The listing builds one solid part. Answer for the finished solid, in the listing's coordinates (mm). A direction names the side the tool comes from. Give positions to 0.01 mm unless a question says otherwise; leave off trailing zeros. Write each loop counter-clockwise with the first axis right and the second up, starting at its lowest first coordinate (ties: lowest second). Pieces come first, ordered by that corner, then holes. Notation, with made-up numbers: (-32, 86) - (20, 86) arc R18 cw to (20, 115) - close; hole circle Ø11 at (-39.5, 65). An arc over 180 degrees is marked (long way). Answer as CSV lines item,"result". Start each with the question number.
(1) Find section B-B (y = 3). Write down the section's boundary in (x, z).
(2) Find section C-C (z = 26.5). Write down the section's boundary in (x, y), then the cut area to 3 significant figures.
(3) For faces 1 (the face through (6.003, 6.459, -38.794)), 2 (the face through (-25, -23, -50)), 3 (the face through (-32.5, -25, 42)), determine the directions among +Z, -Z, +X, -X, +Y, -Y from which every point of the face is accessible in a straight line to the end or side of a thin tool.
(4) Find section D-D (x = -63). Write down the section's boundary in (y, z).
(5) Find section A-A (y = -23.5). State how many separate pieces and enclosed holes the cut face has, then the cut area to 3 significant figures.
(6) Straight lines are drawn through the part: probe 1 along X at (y, z) = (-28, 0); probe 2 along X at (y, z) = (-27, 0); probe 3 along Y at (x, z) = (9, 66.5). For each, find the intervals that lie inside material, in ascending order.
(7) Each of these flat-tipped pins is pushed along its axis until it touches: pin 1 Ø1 at (x, z) = (-4.5, 56.5) entering from -Y; pin 2 Ø3 at (y, z) = (-26.5, -48.5) entering from -X; pin 3 Ø1.5 at (y, z) = (-8.5, -42) entering from -X; pin 4 Ø12 at (x, y) = (-33.5, -6.5) entering from +Z. Where does it stop, or does it pass through?
(8) For a pull along Z with two mould halves and no side action, classify faces 4 (the face through (-27.5, -24, 58)), 5 (the face through (9.415, 2.673, 34.351)), 6 (the face through (-30, -24, -62.5)) as pulls with the +Z half, pulls with the -Z half, needs draft (parallel to the pull), parting line crosses it, or undercut.
from build123d import *

# Parameters (mm, degrees)
SALIENTE_EXTRUIR2_DEPTH             = 75
SALIENTE_EXTRUIR5_DEPTH             = 17
SALIENTE_EXTRUIR5_DIRECTION_2_REACH = 107.612
CROQUIS6_R                          = 3.96875
CORTAR_EXTRUIR2_DEPTH               = 20
CROQUIS16_R                         = 5.96875
CROQUIS16_R_2                       = 3.96875
CORTAR_EXTRUIR3_DEPTH               = 3
CROQUIS17_R                         = 1
CORTAR_EXTRUIR4_DEPTH               = 13


with BuildPart() as part:
    # Croquis1 → Saliente-Extruir2 (new, symmetric)
    with BuildSketch(Plane.XY):
        with BuildLine():
            ThreePointArc((-1.339745962, 5), (12.862399029, 7.937956503), (25, 0))
            Line((25, 0), (0, 0))
            Line((0, 0), (-60.621778265, -35))
            Line((-60.621778265, -35), (-70.621778265, -35))
            Line((-70.621778265, -35), (-1.339745962, 5))
        make_face()
    extrude(amount=SALIENTE_EXTRUIR2_DEPTH, both=True)

    # Croquis3 → Saliente-Extruir5 (add)
    with BuildSketch(Plane.XZ.offset(15)):
        with BuildLine():
            Line((-32.5, 4.330127019), (-32.5, 12.5))
            Line((-32.5, 12.5), (-27.5, 12.5))
            Line((-27.5, 12.5), (-27.5, 4.330127019))
            ThreePointArc((-27.5, 4.330127019), (-25, 0), (-27.5, -4.330127019))
            Line((-27.5, -4.330127019), (-27.5, -12.5))
            Line((-27.5, -12.5), (-32.5, -12.5))
            Line((-32.5, -12.5), (-32.5, -4.330127019))
            ThreePointArc((-32.5, -4.330127019), (-35, 0), (-32.5, 4.330127019))
        make_face()
        with BuildLine():
            Line((-27.5, -45.669872981), (-27.5, -37.5))
            Line((-27.5, -37.5), (-32.5, -37.5))
            Line((-32.5, -37.5), (-32.5, -45.669872981))
            ThreePointArc((-32.5, -45.669872981), (-35, -50), (-32.5, -54.330127019))
            Line((-32.5, -54.330127019), (-32.5, -62.5))
            Line((-32.5, -62.5), (-27.5, -62.5))
            Line((-27.5, -62.5), (-27.5, -54.330127019))
            ThreePointArc((-27.5, -54.330127019), (-25, -50), (-27.5, -45.669872981))
        make_face()
        with BuildLine():
            Line((-27.5, 54.330127019), (-27.5, 62.5))
            Line((-27.5, 62.5), (-32.5, 62.5))
            Line((-32.5, 62.5), (-32.5, 54.330127019))
            ThreePointArc((-32.5, 54.330127019), (-35, 50), (-32.5, 45.669872981))
            Line((-32.5, 45.669872981), (-32.5, 37.5))
            Line((-32.5, 37.5), (-27.5, 37.5))
            Line((-27.5, 37.5), (-27.5, 45.669872981))
            ThreePointArc((-27.5, 45.669872981), (-25, 50), (-27.5, 54.330127019))
        make_face()
    extrude(amount=SALIENTE_EXTRUIR5_DEPTH)

    # Saliente-Extruir5 direction 2: up to this face of the body (flat: up to its plane)
    saliente_extruir5_direction_2_end = Plane(part.part.faces().sort_by_distance((-30.310889132, -17.5, 0))[0])
    # Croquis3 → Saliente-Extruir5 direction 2 (add, up to the picked face)
    with BuildSketch(Plane.XZ.offset(15), mode=Mode.PRIVATE) as saliente_extruir5_direction_2_sk1:
        with BuildLine():
            Line((-32.5, 4.330127019), (-32.5, 12.5))
            Line((-32.5, 12.5), (-27.5, 12.5))
            Line((-27.5, 12.5), (-27.5, 4.330127019))
            ThreePointArc((-27.5, 4.330127019), (-25, 0), (-27.5, -4.330127019))
            Line((-27.5, -4.330127019), (-27.5, -12.5))
            Line((-27.5, -12.5), (-32.5, -12.5))
            Line((-32.5, -12.5), (-32.5, -4.330127019))
            ThreePointArc((-32.5, -4.330127019), (-35, 0), (-32.5, 4.330127019))
        make_face()
    saliente_extruir5_direction_2_tool1 = split(extrude(saliente_extruir5_direction_2_sk1.sketch, amount=-SALIENTE_EXTRUIR5_DIRECTION_2_REACH, mode=Mode.PRIVATE), bisect_by=saliente_extruir5_direction_2_end, keep=Keep.BOTH, mode=Mode.PRIVATE)
    # Croquis3 → Saliente-Extruir5 direction 2 (add, up to the picked face)
    with BuildSketch(Plane.XZ.offset(15), mode=Mode.PRIVATE) as saliente_extruir5_direction_2_sk2:
        with BuildLine():
            Line((-27.5, -45.669872981), (-27.5, -37.5))
            Line((-27.5, -37.5), (-32.5, -37.5))
            Line((-32.5, -37.5), (-32.5, -45.669872981))
            ThreePointArc((-32.5, -45.669872981), (-35, -50), (-32.5, -54.330127019))
            Line((-32.5, -54.330127019), (-32.5, -62.5))
            Line((-32.5, -62.5), (-27.5, -62.5))
            Line((-27.5, -62.5), (-27.5, -54.330127019))
            ThreePointArc((-27.5, -54.330127019), (-25, -50), (-27.5, -45.669872981))
        make_face()
    saliente_extruir5_direction_2_tool2 = split(extrude(saliente_extruir5_direction_2_sk2.sketch, amount=-SALIENTE_EXTRUIR5_DIRECTION_2_REACH, mode=Mode.PRIVATE), bisect_by=saliente_extruir5_direction_2_end, keep=Keep.BOTH, mode=Mode.PRIVATE)
    # Croquis3 → Saliente-Extruir5 direction 2 (add, up to the picked face)
    with BuildSketch(Plane.XZ.offset(15), mode=Mode.PRIVATE) as saliente_extruir5_direction_2_sk3:
        with BuildLine():
            Line((-27.5, 54.330127019), (-27.5, 62.5))
            Line((-27.5, 62.5), (-32.5, 62.5))
            Line((-32.5, 62.5), (-32.5, 54.330127019))
            ThreePointArc((-32.5, 54.330127019), (-35, 50), (-32.5, 45.669872981))
            Line((-32.5, 45.669872981), (-32.5, 37.5))
            Line((-32.5, 37.5), (-27.5, 37.5))
            Line((-27.5, 37.5), (-27.5, 45.669872981))
            ThreePointArc((-27.5, 45.669872981), (-25, 50), (-27.5, 54.330127019))
        make_face()
    saliente_extruir5_direction_2_tool3 = split(extrude(saliente_extruir5_direction_2_sk3.sketch, amount=-SALIENTE_EXTRUIR5_DIRECTION_2_REACH, mode=Mode.PRIVATE), bisect_by=saliente_extruir5_direction_2_end, keep=Keep.BOTH, mode=Mode.PRIVATE)
    add(saliente_extruir5_direction_2_tool1.solids().sort_by(Axis((-30, -15, 0), (0, 1, 0)))[0])
    add(saliente_extruir5_direction_2_tool2.solids().sort_by(Axis((-30, -15, -50), (0, 1, 0)))[0])
    add(saliente_extruir5_direction_2_tool3.solids().sort_by(Axis((-30, -15, 50), (0, 1, 0)))[0])

    # Croquis6 → Cortar-Extruir2 (cut)
    with BuildSketch(Plane(origin=(0, 8.271300641, 0), x_dir=(1, 0, 0), z_dir=(0, 1, 0))):
        with Locations(Location((11.830127019, 37.5, 0), (0, 0, 270))):
            Circle(CROQUIS6_R)
        with Locations(Location((11.830127019, -37.5, 0), (0, 0, 270))):
            Circle(CROQUIS6_R)
    extrude(amount=-CORTAR_EXTRUIR2_DEPTH, mode=Mode.SUBTRACT)

    # Croquis16 → Cortar-Extruir3 (cut)
    # profile 1 of 2: a face of its own
    with BuildSketch(Plane(origin=(0, 8.271300641, 0), x_dir=(1, 0, 0), z_dir=(0, 1, 0))):
        with Locations(Location((11.830127019, 37.5, 0), (0, 0, 270))):
            Circle(CROQUIS16_R)
        with Locations(Location((11.830127019, 37.5, 0), (0, 0, 270))):
            Circle(CROQUIS16_R_2, mode=Mode.SUBTRACT)
    # profile 2 of 2: a face of its own
    with BuildSketch(Plane(origin=(0, 8.271300641, 0), x_dir=(1, 0, 0), z_dir=(0, 1, 0))):
        with Locations(Location((11.830127019, -37.5, 0), (0, 0, 270))):
            Circle(CROQUIS16_R)
        with Locations(Location((11.830127019, -37.5, 0), (0, 0, 270))):
            Circle(CROQUIS16_R_2, mode=Mode.SUBTRACT)
    extrude(amount=-CORTAR_EXTRUIR3_DEPTH, mode=Mode.SUBTRACT)

    # Croquis17 → Cortar-Extruir4 (cut)
    with BuildSketch(Plane.XZ.offset(32)):
        with Locations(Location((-30, 50, 0), (0, 0, 270))):
            Circle(CROQUIS17_R)
        with Locations(Location((-30, 0, 0), (0, 0, 270))):
            Circle(CROQUIS17_R)
        with Locations(Location((-30, -50, 0), (0, 0, 270))):
            Circle(CROQUIS17_R)
    extrude(amount=-CORTAR_EXTRUIR4_DEPTH, mode=Mode.SUBTRACT)


solid = part.part
Result set:
1,outline,"(-4.8, -75) - (22.45, -75) - (22.45, 75) - (-4.8, 75) - close; hole circle Ø7.94 at (11.83, -37.5); hole circle Ø7.94 at (11.83, 37.5)"
2,outline,"(-70.62, -35) - (-60.62, -35) - (0, 0) - (25, 0) arc R19 ccw to (-1.34, 5) - close"
2,area,"540 mm^2"
3,face 1,"+Y"
3,face 2,"+X, -Y"
3,face 3,"-Y"
4,outline,"(-35, -75) - (-30.6, -75) - (-30.6, 75) - (-35, 75) - close"
5,separate pieces,"4"
5,enclosed holes,"3"
5,area,"1,960 mm^2"
6,probe 1,"-58.5 to -48.5, -35 to -31, -29 to -25"
6,probe 2,"-56.77 to -46.77, -35 to -31, -29 to -25"
6,probe 3,"0 to 8.27"
7,pin 1,"y = -2.89"
7,pin 2,"x = -58.5"
7,pin 3,"x = -26.02"
7,pin 4,"through"
8,face 4,"needs draft"
8,face 5,"undercut"
8,face 6,"pulls with the -Z half"
